from build123d import *

# Parameters (mm, degrees)
SKETCH_1_W                   = 30
SKETCH_1_H                   = 30
EXTRUDE_1_DEPTH              = 30
SKETCH_2_R                   = 4
CUT_EXTRUDE_1_DEPTH          = 30
SKETCH_3_W                   = 30
SKETCH_3_H                   = 10
EXTRUDE_2_DEPTH              = 30
SKETCH_4_W                   = 30
SKETCH_4_H                   = 10
EXTRUDE_3_DEPTH              = 30
HOLE_WIZARD_M4_1_D           = 4.5
HOLE_WIZARD_M4_1_CBORE_D     = 10
HOLE_WIZARD_M4_1_CBORE_DEPTH = 4


with BuildPart() as part:
    # 스케치1 → 보스-돌출1 (new body)
    with BuildSketch(Plane.XY):
        Rectangle(SKETCH_1_W, SKETCH_1_H)
    extrude(amount=EXTRUDE_1_DEPTH)

    # 스케치2 → 컷-돌출1 (cut)
    with BuildSketch(Plane.XY.offset(30)):
        Circle(SKETCH_2_R)
    extrude(amount=-CUT_EXTRUDE_1_DEPTH, mode=Mode.SUBTRACT)

    # 스케치3 → 보스-돌출2 (add)
    with BuildSketch(Plane(origin=(15, 0, 0), x_dir=(0, 0, -1), z_dir=(1, 0, 0))):
        with Locations((-15, 10)):
            Rectangle(SKETCH_3_W, SKETCH_3_H)
    extrude(amount=EXTRUDE_2_DEPTH)

    # 스케치4 → 보스-돌출3 (add)
    with BuildSketch(Plane.ZY.offset(15)):
        with Locations((15, 10)):
            Rectangle(SKETCH_4_W, SKETCH_4_H)
    extrude(amount=EXTRUDE_3_DEPTH)

    # M4 소켓 머리 캡 나사용 카운터보어1 (through all)
    with Locations(Plane(origin=(0, 5, 0), x_dir=(-1, 0, 0), z_dir=(0, -1, 0))):
        with Locations((-30, -15), (30, -15)):
            CounterBoreHole(HOLE_WIZARD_M4_1_D / 2, HOLE_WIZARD_M4_1_CBORE_D / 2, HOLE_WIZARD_M4_1_CBORE_DEPTH)


solid = part.part
Model file for the job. Use its own axes, mm. A direction names the side the tool comes from. Round coordinates to 2 decimals unless told otherwise and drop trailing zeros. Loops run counter-clockwise (first coordinate to the right, second up) from the corner with the lowest first, then second, coordinate; pieces in that order, holes last. Notation, with made-up numbers: (27, -40) -> (78, -40) arc R21 ccw to (78, -25) -> close; hole circle Ø7 at (5.25, 80). An arc over 180 degrees is marked (long way). Answer as CSV lines item,"result". Start each with the question number.
1) Probe line 1 along X through (y, z) = (12.7, 15); line 2 along Z through (x, y) = (-30, 13.1); line 3 along Z through (x, y) = (-30, 6.75). List the from-to ranges inside material, lowest first.
2) Slice it at B-B (y = 0). List the corners of the cut face in (x, z), plus the area to 3 significant figures.
3) Slice it at A-A (z = 15). List the corners of the cut face in (x, y).
4) Slice it at C-C (x = -30). List the corners of the cut face in (y, z), plus the area to 3 significant figures.
5) Pin check, flat tips, straight feed: P1, Ø4, axis at x = 26, z = 15, coming from the -Y side; P2, Ø16, axis at y = -4.5, z = 14.5, coming from the +X side; P3, Ø5, axis at x = 32, z = 15, coming from the -Y side. Stop position of each tip, or through.
6) Tool access for faces 1 (the face through (15, -5, 15)), 2 (the face through (29, 9, 17.2)), 3 (the face through (-15, -5, 15)), 4 (the face through (45, 10, 15)), 5 (the face through (1, 15, 15)): list every direction of +Z, -Z, +X, -X, +Y, -Y with a clear straight run to the whole face (end or side of a thin tool).
7) Mould opens along Z. For faces 6 (the face through (32.08, 12.04, 15.86)), 7 (the face through (1, 6, 30)), 8 (the face through (-26, 5, 11)) say: +Z half, -Z half, draft (parallel to the pull), parting line (faces both ways), or undercut.
8) Slice it at D-D (z = 26.5). List the corners of the cut face in (x, y).
Filled in:
1,line 1,"x = -45 to -32.25, -27.75 to 27.75, 32.25 to 45"
1,line 2,"z = 0 to 12.75, 17.25 to 30"
1,line 3,"z = 0 to 10, 20 to 30"
2,outline,"(-15, 0) -> (-4, 0) -> (-4, 30) -> (-15, 30) -> close; (4, 0) -> (15, 0) -> (15, 30) -> (4, 30) -> close"
2,area,"660 mm2"
3,outline,"(-45, 5) -> (-35, 5) -> (-35, 9) -> (-32.25, 9) -> (-32.25, 15) -> (-45, 15) -> close; (-27.75, 9) -> (-25, 9) -> (-25, 5) -> (-15, 5) -> (-15, -15) -> (15, -15) -> (15, 5) -> (25, 5) -> (25, 9) -> (27.75, 9) -> (27.75, 15) -> (-27.75, 15) -> close; (32.25, 9) -> (35, 9) -> (35, 5) -> (45, 5) -> (45, 15) -> (32.25, 15) -> close; hole circle Ø8 at (0, 0)"
4,outline,"(5, 0) -> (15, 0) -> (15, 12.75) -> (9, 12.75) -> (9, 10) -> (5, 10) -> close; (5, 20) -> (9, 20) -> (9, 17.25) -> (15, 17.25) -> (15, 30) -> (5, 30) -> close"
4,area,"233 mm2"
5,P1,"stops at y = 5"
5,P2,"stops at x = 15"
5,P3,"stops at y = 9"
6,face 1,"+Z, -Z, +X, -Y"
6,face 2,"-Y"
6,face 3,"+Z, -Z, -X, -Y"
6,face 4,"+Z, -Z, +X, +Y, -Y"
6,face 5,"+Z, -Z, +X, -X, +Y"
7,face 6,"undercut"
7,face 7,"+Z half"
7,face 8,"draft"
8,outline,"(-45, 5) -> (-15, 5) -> (-15, -15) -> (15, -15) -> (15, 5) -> (45, 5) -> (45, 15) -> (-45, 15) -> close; hole circle Ø8 at (0, 0)"
